from build123d import *

# Parameters (mm, degrees)
F0_W     = 20
F0_H     = 20
F1_DEPTH = 30
F2_R     = 4
F3_DEPTH = 25
F4_SIZE  = 9.99999


# Not quite as in the source:
# - a fillet or chamfer is up to 0.001 mm smaller than in the source, because OpenCascade refuses the exact size


with BuildPart() as f1:
    # F0 (on Top) → F1 (new body)
    with BuildSketch(Plane.XY):
        Rectangle(F0_W, F0_H)
    extrude(amount=F1_DEPTH)

    # F2 (on face) → F3 (join)
    with BuildSketch(Plane.XY.offset(30)):
        Circle(F2_R)
    extrude(amount=F3_DEPTH)

    # F4 (size 10 in the source; OpenCascade refuses exactly that, so slightly less here)
    f4_edges = [f1.edges().sort_by_distance(p)[0] for p in [
        (10, 0, 0),
        (0, 10, 0),
        (-10, 0, 0),
        (0, -10, 0),
    ]]
    chamfer(f4_edges, length=F4_SIZE)


solid = f1.part
Work out the finished part from the listing and answer in its coordinate system (mm). A direction names the side the tool comes from. Give positions to 0.01 mm unless a question says otherwise; leave off trailing zeros. Write each loop counter-clockwise with the first axis right and the second up, starting at its lowest first coordinate (ties: lowest second). Pieces come first, ordered by that corner, then holes.
Q1. Straight lines are drawn through the part: L1, parallel to Z at x = 1.5, y = 3.5; L2, parallel to Z at x = 4.75, y = 3.25; L3, parallel to Y at x = -3, z = 38. For each, find the intervals that lie inside material, in ascending order.
Answer:
L1: z = 3.5 to 55
L2: z = 4.75 to 30
L3: y = -2.65 to 2.65
Q2. The part is cut by section C-C on y = 8.5. Give the vertices of the cut face in (x, z), and give its area (3 significant figures).
Answer:
outline: (-10, 10) - (-8.5, 8.5) - (8.5, 8.5) - (10, 10) - (10, 30) - (-10, 30) - close
area: 428 mm2
Q3. A tool of negligible diameter and unlimited length cuts with its end or side. For faces 1 (the face through (4.3, 0.1, 30)), 2 (the face through (0, 10, 20)), from which of +Z, -Z, +X, -X, +Y, -Y can it reach the whole face along a straight path? Write none if from no direction.
Answer:
face 1: +Z
face 2: +Z, -Z, +X, -X, +Y
Q4. The part is cut by section A-A on x = -8. Give the vertices of the cut face in (y, z), and give its area (3 significant figures).
Answer:
outline: (-10, 10) - (-8, 8) - (8, 8) - (10, 10) - (10, 30) - (-10, 30) - close
area: 436 mm2
Q5. The part is cut by section B-B on z = 46. Give the vertices of the cut face in (x, y), and give its area (3 significant figures).
Answer:
outline: circle Ø8 at (0, 0)
area: 50.3 mm2
Q6. Given pin 1 (4 mm diameter, centred on x = -5.5, z = 39.5, fed in from +Y); pin 2 (3 mm diameter, centred on x = -6, y = -6, fed in from +Z); pin 3 (3 mm diameter, centred on x = -2.5, z = 33, fed in from +Y); pin 4 (12 mm diameter, centred on y = -1.5, z = 9, fed in from -X), each flat-ended and moving along its own axis, determine where each tip first touches the part or whether it passes through.
Answer:
pin 1: stops at y = 1.94
pin 2: stops at z = 30
pin 3: stops at y = 3.87
pin 4: stops at x = -10
